Autodesk Inventor part; units mm, degrees
ref_plane "YZ Plane" through (0, 0, 0) normal (1, 0, 0) x (0, 1, 0)
ref_plane "XZ Plane" through (0, 0, 0) normal (0, 1, 0) x (-1, 0, 0)
ref_plane "XY Plane" through (0, 0, 0) normal (0, 0, 1) x (1, 0, 0)
sketch "Sketch1" plane through (0, 0, 0) normal (0, 1, 0) x (-1, 0, 0)
  circle A0 centre (0, 0) radius 3
  dimension "d0" = 6
extrude "Extrusion1" add sketch "Sketch1" along normal blind 15.9
chamfer "Chamfer1" distance 0.5 angle 45 1 edges at (3, 15.9, 0)
chamfer "Chamfer2" distance 0.5 angle 45 1 edges at (3, 0, 0)
thread "Thread1"
properties part number "din m6-10 Flat point socket set screw"
Check sheet for the modelled part. Datum: model origin and axes. Units: mm. Give positions to 0.01 mm unless a question says otherwise; leave off trailing zeros. Order: outer loops, then holes, each group sorted by start corner. A loop starts at its lowest first (then second) coordinate and runs counter-clockwise, first axis right, second up. Notation, with made-up numbers: (1, -39) -> (29, -39) arc R20 ccw to (29, -1) -> close; hole circle Ø4 at (17.25, 47.25). An arc over 180 degrees is marked (long way). Return JSON: item names as keys, results as strings.
1. Cross-section at A-A, the plane y = 11.5. Record the cut outline in (x, z), plus the area to 3 significant figures.
From the geometry:
{"outline": "circle Ø6 at (0, 0)", "area": "28.3 mm^2"}
2. Material ranges on probe 1 along Z at (x, y) = (-0.15, 8); probe 2 along X at (y, z) = (9, 1.4), recorded low to high. Write a range as [from, to].
From the geometry:
{"probe 1": "[-3, 3]", "probe 2": "[-2.65, 2.65]"}
3. Go/stop test with a flat-tipped pin: P1, Ø1.5, axis at x = -1, y = 3.5, coming from the -Z side. Record where the tip stops, or that it passes through.
From the geometry:
{"P1": "z = -2.99"}
